Design review of the part built by this model. Coordinates are the model's own, in mm. Coordinates: 2 decimals unless noted, no trailing zeros. Loops run counter-clockwise (first coordinate to the right, second up) from the corner with the lowest first, then second, coordinate; pieces in that order, holes last.
Q1. Add section C-C on x = -12.7. Give the boundary of the cut face in (y, z).
Q2. Add section A-A on x = -63.5. Give the boundary of the cut face in (y, z), and give its area (3 significant figures).
Q3. Wall thickness on probe 1 along Z at (x, y) = (-12.7, 3.1); probe 2 along X at (y, z) = (4.35, -14); probe 3 along X at (y, z) = (3.1, -29): over which ranges is each line inside the solid? List them lowest first.
Q4. Add section B-B on z = -63.5. Give the boundary of the cut face in (x, y), and give its area (3 significant figures).
Q5. For P1, Ø1.2, axis at y = 3, z = -31, coming from the -X side; P2, Ø2, axis at y = 1.5, z = -22.5, coming from the +X side; P3, Ø2.5, axis at y = 1.5, z = -66.5, coming from the -X side; P4, Ø1.5, axis at y = 1.5, z = -50, coming from the -X side, all flat-tipped, find the tip position at first contact; note any pin that passes through.
Q6. Add section D-D on y = 1.7. Give the number of separate pieces and of enclosed holes in the cut face, and give its area (3 significant figures).
Autodesk Inventor part; units mm, degrees
ref_plane "YZ Plane" through (0, 0, 0) normal (1, 0, 0) x (0, 1, 0)
ref_plane "XZ Plane" through (0, 0, 0) normal (0, 1, 0) x (-1, 0, 0)
ref_plane "XY Plane" through (0, 0, 0) normal (0, 0, 1) x (1, 0, 0)
sketch "Sketch1" plane through (0, 0, 0) normal (0, 1, 0) x (-1, 0, 0)
  line L0 (0, -11.8745) -> (0, -71.4375)
  line L1 (4.7625, -76.2) -> (20.6375, -76.2)
  line L2 (76.2, -20.6375) -> (76.2, -11.8745)
  line L3 (71.4375, -7.112) -> (4.7625, -7.112)
  circle A0 centre (12.7, -38.1) radius 2.54
  arc A1 (4.7625, -7.112) -> (0, -11.8745) centre (4.7625, -11.8745) ccw
  circle A2 centre (12.7, -50.8) radius 2.54
  circle A3 centre (12.7, -63.5) radius 2.54
  circle A4 centre (38.1, -12.7) radius 2.54
  circle A5 centre (50.8, -12.7) radius 2.54
  circle A6 centre (63.5, -12.7) radius 2.54
  line L4 (14.4961, -61.7039) -> (61.7039, -14.4961) construction
  line L5 (26.7949, -56.1403) -> (56.1403, -26.7949)
  line L6 (33.5301, -35.9347) -> (35.9347, -33.5301)
  line L7 (25.4, -76.2) -> (25.4, -25.4) construction
  line L8 (76.2, -25.4) -> (25.4, -25.4) construction
  line L9 (25.4, -59.5079) -> (25.4, -71.4375)
  line L10 (71.4375, -25.4) -> (59.5079, -25.4)
  arc A7 (71.4375, -25.4) -> (76.2, -20.6375) centre (71.4375, -20.6375) ccw
  arc A8 (76.2, -11.8745) -> (71.4375, -7.112) centre (71.4375, -11.8745) ccw
  arc A9 (20.6375, -76.2) -> (25.4, -71.4375) centre (20.6375, -71.4375) ccw
  arc A10 (0, -71.4375) -> (4.7625, -76.2) centre (4.7625, -71.4375) ccw
  line L11 (32.5671, -25.4) -> (30.1625, -25.4)
  line L12 (25.4, -32.5671) -> (25.4, -30.1625)
  arc A11 (59.5079, -25.4) -> (56.1403, -26.7949) centre (59.5079, -30.1625) ccw
  arc A12 (26.7949, -56.1403) -> (25.4, -59.5079) centre (30.1625, -59.5079) ccw
  arc A13 (35.9347, -33.5301) -> (32.5671, -25.4) centre (32.5671, -30.1625) ccw
  arc A14 (25.4, -32.5671) -> (33.5301, -35.9347) centre (30.1625, -32.5671) ccw
  arc A15 (30.1625, -25.4) -> (25.4, -30.1625) centre (30.1625, -30.1625) ccw
  point P0 (0, 0)
  point P1 (0, -76.2)
  point P2 (25.4, -57.5352)
  point P3 (57.5352, -25.4)
  point P4 (25.4, -44.0648)
  point P5 (44.0648, -25.4)
  dimension "d2" = 76.2
  dimension "d4" = 5.08
  dimension "d5" = 4.7625
  dimension "d7" = 12.7
  dimension "d8" = 12.7
  dimension "d9" = 12.7
  dimension "d10" = 5.08
  dimension "d11" = 12.7
  dimension "d12" = 12.7
  dimension "d13" = 38.1
  dimension "d18" = 25.4
  dimension "d20" = 4.7625
  dimension "d21" = 4.7625
  dimension "d22" = 4.7625
  dimension "d23" = 4.7625
  dimension "d24" = 4.7625
  dimension "d29" = 18.288
  dimension "d30" = 25.4
  dimension "d31" = 76.2
  dimension "d32" = 12.7
  dimension "d33" = 38.1
extrude "Extrusion1" add sketch "Sketch1" along normal blind 4.7625
sketch "Sketch2" plane through (0, 4.7625, 0) normal (0, 1, 0) x (1, 0, 0)
  line L0 (-71.4375, 7.112) -> (-4.7625, 7.112)
  line L1 (-76.2, 8.382) -> (0, 8.382)
  line L2 (-76.2, 20.6375) -> (-76.2, 11.8745)
  line L3 (0, 11.8745) -> (0, 71.4375)
  line L4 (-4.7625, 7.112) -> (0, 7.112)
  line L5 (0, 7.112) -> (0, 8.382)
  line L6 (-76.2, 8.382) -> (-76.2, 7.112)
  line L7 (-76.2, 7.112) -> (-71.4375, 7.112)
  point P0 (0, 0)
  dimension "d34" = 1.27
extrude "Extrusion2" cut sketch "Sketch2" against normal through all
fillet "Fillet1" radius 4.7752 2 edges at (-74.6754, 2.3813, -8.382) (-1.5246, 2.3813, -8.382)
properties part number "ELEV_007_SUPBRK2" material "Aluminum 6061"
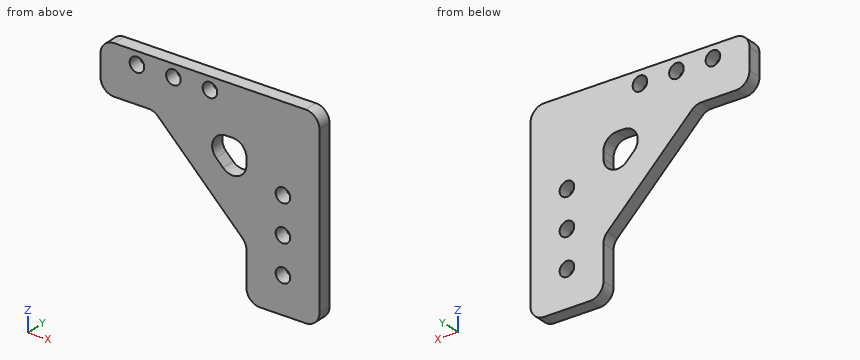
Entries:
1. outline: (0, -76.2) - (4.76, -76.2) - (4.76, -66.04) - (0, -66.04) - close; (0, -60.96) - (4.76, -60.96) - (4.76, -53.34) - (0, -53.34) - close; (0, -48.26) - (4.76, -48.26) - (4.76, -40.64) - (0, -40.64) - close; (0, -35.56) - (4.76, -35.56) - (4.76, -8.38) - (0, -8.38) - close
2. outline: (0, -25.4) - (4.76, -25.4) - (4.76, -15.24) - (0, -15.24) - close; (0, -10.16) - (4.76, -10.16) - (4.76, -8.38) - (0, -8.38) - close
2. area: 56.9 mm2
3. probe 1: z = -76.2 to -66.04, -60.96 to -53.34, -48.26 to -40.64, -35.56 to -8.38
3. probe 2: x = -76.2 to -65.68, -61.32 to -52.98, -48.62 to -40.28, -35.92 to 0
3. probe 3: x = -53.94 to -37.19, -25.54 to 0
4. outline: (-25.4, 0) - (-15.24, 0) - (-15.24, 4.76) - (-25.4, 4.76) - close; (-10.16, 0) - (0, 0) - (0, 4.76) - (-10.16, 4.76) - close
4. area: 96.8 mm2
5. P1: stops at x = -52.54
5. P2: stops at x = 0
5. P3: stops at x = -25.4
5. P4: stops at x = -33.69
6. separate pieces: 1
6. enclosed holes: 7
6. area: 2,850 mm2
